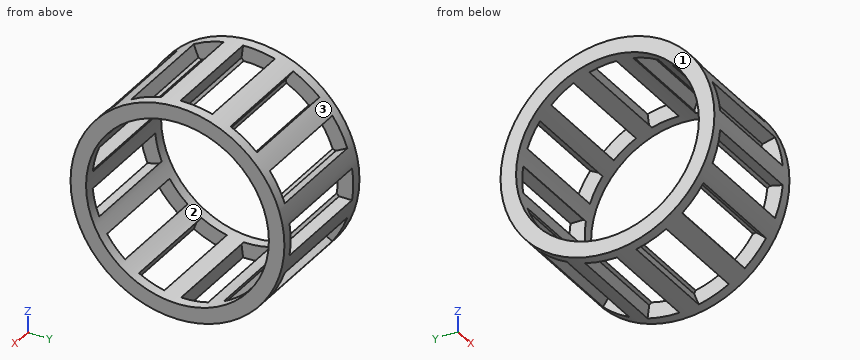
from build123d import *

# Parameters (mm, degrees)
SCHIZZO4_W                  = 12
SCHIZZO4_H                  = 1.45
TAGLIO_ESTRUSIONE1_DEPTH    = 5
RIPETIZIONECIRCOLARE1_COUNT = 13


with BuildPart() as part:
    # Schizzo4 → Rivoluzione1 (revolve)
    with BuildSketch(Plane.XY):
        with Locations((0, 9.275)):
            Rectangle(SCHIZZO4_W, SCHIZZO4_H)
    revolve(axis=Axis((0, 0, 0), (-1, 0, 0)))

    # Schizzo6 → Taglio-Estrusione1 (cut, symmetric)
    with BuildSketch(Plane(origin=(0, 0, 0), x_dir=(0, 0, -1), z_dir=(1, 0, 0))):
        with BuildLine():
            Line((-1.5, 10), (-1.5, 8.677124344))
            ThreePointArc((-1.5, 8.677124344), (0, 8), (1.5, 8.677124344))
            Line((1.5, 8.677124344), (1.5, 10))
            ThreePointArc((1.5, 10), (0, 11.5), (-1.5, 10))
        make_face()
    taglio_estrusione1 = extrude(amount=TAGLIO_ESTRUSIONE1_DEPTH, both=True, mode=Mode.SUBTRACT)

    # RipetizioneCircolare1: Taglio-Estrusione1 ×13 about axis
    ripetizionecircolare1_axis = Axis((0, 0, 0), (1, 0, 0))
    for i in range(1, RIPETIZIONECIRCOLARE1_COUNT):
        add(taglio_estrusione1.rotate(ripetizionecircolare1_axis, i * 360 / RIPETIZIONECIRCOLARE1_COUNT), mode=Mode.SUBTRACT)


solid = part.part
Build history of the part. All positions in model axes, mm. Face numbers are marked on the shaded views. Give positions to 0.01 mm unless a question says otherwise; leave off trailing zeros. Write each loop counter-clockwise with the first axis right and the second up, starting at its lowest first coordinate (ties: lowest second). Pieces come first, ordered by that corner, then holes. Notation, with made-up numbers: (57, 26.5) - (86, 26.5) arc R4 cw to (86, 32.5) - close; hole circle Ø5 at (-33, -10.75). An arc over 180 degrees is marked (long way). Use one line per item in the form item = value. Start each with the question number.
1. Two-plate mould, pull along Z, no slides. Class the marked faces 1, 2 and 3: released by +Z, released by -Z, zero draft, split by the parting line, or undercut.
2. Band-saw the part on A-A on z = 0. Write the cut outline in (x, y).
3. Band-saw the part on B-B on x = 2.5. Count the separate pieces of the cut face and the enclosed holes in it, plus the area to 3 significant figures.
4. Drop flat-ended pins along their axis: pin 1 Ø3 at (x, z) = (1.5, -3.5) entering from +Y; pin 2 Ø0.6 at (x, y) = (-2, 9) entering from +Z; pin 3 Ø4 at (x, y) = (1.5, -4.5) entering from +Z. Give the stop position or say it passes through.
5. Probe line 1 (X direction, y = 8.25, z = 5.5); line 2 (Y direction, x = -2, z = -0.25); line 3 (Y direction, x = -4.5, z = -6.75). List the from-to ranges inside material, lowest first. Write a range as [from, to].
Conclusion:
q1.face_1 = zero draft
q1.face_2 = undercut
q1.face_3 = split by the parting line
q2.outline = (-6, -10) - (6, -10) - (6, -8.55) - (-6, -8.55) - close; (-6, 8.55) - (-5, 8.55) - (-5, 10) - (-6, 10) - close; (5, 8.55) - (6, 8.55) - (6, 10) - (5, 10) - close
q3.separate_pieces = 13
q3.enclosed_holes = 0
q3.area = 28.4 mm²
q4.pin_1 = 9.8
q4.pin_2 = 3.19
q4.pin_3 = 8.71
q5.line_1 = [-6, -5], [5, 6]
q5.line_2 = [-10, -8.55]
q5.line_3 = [-5.49, -5.25], [6.48, 7.38]
